from build123d import *

# Parameters (mm, degrees)
F0_W     = 3
F0_H     = 27
F1_DEPTH = 2


with BuildPart() as f1:
    # F0 (on Top) → F1 (new body)
    with BuildSketch(Plane.XY):
        with Locations((-86.87473, 11.051753)):
            Rectangle(F0_W, F0_H)
        with Locations((-82.87473, 11.051753)):
            Rectangle(F0_W, F0_H)
        with Locations((-78.87473, 11.051753)):
            Rectangle(F0_W, F0_H)
        with Locations((-74.87473, 11.051753)):
            Rectangle(F0_W, F0_H)
        with Locations((-70.87473, 11.051753)):
            Rectangle(F0_W, F0_H)
        with Locations((-66.87473, 11.051753)):
            Rectangle(F0_W, F0_H)
        with Locations((-62.87473, 11.051753)):
            Rectangle(F0_W, F0_H)
        with Locations((-58.87473, 11.051753)):
            Rectangle(F0_W, F0_H)
        with Locations((-54.87473, 11.051753)):
            Rectangle(F0_W, F0_H)
        with Locations((-50.87473, 11.051753)):
            Rectangle(F0_W, F0_H)
        with Locations((-46.87473, 11.051753)):
            Rectangle(F0_W, F0_H)
        with Locations((-42.87473, 11.051753)):
            Rectangle(F0_W, F0_H)
        with Locations((-38.87473, 11.051753)):
            Rectangle(F0_W, F0_H)
        with Locations((-34.87473, 11.051753)):
            Rectangle(F0_W, F0_H)
        with Locations((-30.87473, 11.051753)):
            Rectangle(F0_W, F0_H)
        with Locations((-26.87473, 11.051753)):
            Rectangle(F0_W, F0_H)
        with Locations((-22.87473, 11.051753)):
            Rectangle(F0_W, F0_H)
        with Locations((-18.87473, 11.051753)):
            Rectangle(F0_W, F0_H)
        with Locations((-14.87473, 11.051753)):
            Rectangle(F0_W, F0_H)
        with Locations((-10.87473, 11.051753)):
            Rectangle(F0_W, F0_H)
        with Locations((-6.87473, 11.051753)):
            Rectangle(F0_W, F0_H)
        with Locations((-2.87473, 11.051753)):
            Rectangle(F0_W, F0_H)
        with Locations((1.12527, 11.051753)):
            Rectangle(F0_W, F0_H)
        with Locations((5.12527, 11.051753)):
            Rectangle(F0_W, F0_H)
        with Locations((9.12527, 11.051753)):
            Rectangle(F0_W, F0_H)
        with Locations((13.12527, 11.051753)):
            Rectangle(F0_W, F0_H)
        with Locations((17.12527, 11.051753)):
            Rectangle(F0_W, F0_H)
        with Locations((21.12527, 11.051753)):
            Rectangle(F0_W, F0_H)
        with Locations((25.12527, 11.051753)):
            Rectangle(F0_W, F0_H)
        with Locations((29.12527, 11.051753)):
            Rectangle(F0_W, F0_H)
        with Locations((33.12527, 11.051753)):
            Rectangle(F0_W, F0_H)
        with Locations((37.12527, 11.051753)):
            Rectangle(F0_W, F0_H)
        with Locations((41.12527, 11.051753)):
            Rectangle(F0_W, F0_H)
        with Locations((45.12527, 11.051753)):
            Rectangle(F0_W, F0_H)
        with Locations((49.12527, 11.051753)):
            Rectangle(F0_W, F0_H)
        with Locations((53.12527, 11.051753)):
            Rectangle(F0_W, F0_H)
        with Locations((57.12527, 11.051753)):
            Rectangle(F0_W, F0_H)
        with Locations((61.12527, 11.051753)):
            Rectangle(F0_W, F0_H)
        with Locations((65.12527, 11.051753)):
            Rectangle(F0_W, F0_H)
        with Locations((69.12527, 11.051753)):
            Rectangle(F0_W, F0_H)
        with Locations((73.12527, 11.051753)):
            Rectangle(F0_W, F0_H)
        with Locations((77.12527, 11.051753)):
            Rectangle(F0_W, F0_H)
        with Locations((81.12527, 11.051753)):
            Rectangle(F0_W, F0_H)
        with Locations((85.12527, 11.051753)):
            Rectangle(F0_W, F0_H)
        Polygon((86.62527, 37.551753), (-88.37473, 37.551753), (-88.37473, 24.551753), (-85.37473, 24.551753), (-84.37473, 24.551753), (-81.37473, 24.551753), (-80.37473, 24.551753), (-77.37473, 24.551753), (-76.37473, 24.551753), (-73.37473, 24.551753), (-72.37473, 24.551753), (-69.37473, 24.551753), (-68.37473, 24.551753), (-65.37473, 24.551753), (-64.37473, 24.551753), (-61.37473, 24.551753), (-60.37473, 24.551753), (-57.37473, 24.551753), (-56.37473, 24.551753), (-53.37473, 24.551753), (-52.37473, 24.551753), (-49.37473, 24.551753), (-48.37473, 24.551753), (-45.37473, 24.551753), (-44.37473, 24.551753), (-41.37473, 24.551753), (-40.37473, 24.551753), (-37.37473, 24.551753), (-36.37473, 24.551753), (-33.37473, 24.551753), (-32.37473, 24.551753), (-29.37473, 24.551753), (-28.37473, 24.551753), (-25.37473, 24.551753), (-24.37473, 24.551753), (-21.37473, 24.551753), (-20.37473, 24.551753), (-17.37473, 24.551753), (-16.37473, 24.551753), (-13.37473, 24.551753), (-12.37473, 24.551753), (-9.37473, 24.551753), (-8.37473, 24.551753), (-5.37473, 24.551753), (-4.37473, 24.551753), (-1.37473, 24.551753), (-0.37473, 24.551753), (2.62527, 24.551753), (3.62527, 24.551753), (6.62527, 24.551753), (7.62527, 24.551753), (10.62527, 24.551753), (11.62527, 24.551753), (14.62527, 24.551753), (15.62527, 24.551753), (18.62527, 24.551753), (19.62527, 24.551753), (22.62527, 24.551753), (23.62527, 24.551753), (26.62527, 24.551753), (27.62527, 24.551753), (30.62527, 24.551753), (31.62527, 24.551753), (34.62527, 24.551753), (35.62527, 24.551753), (38.62527, 24.551753), (39.62527, 24.551753), (42.62527, 24.551753), (43.62527, 24.551753), (46.62527, 24.551753), (47.62527, 24.551753), (50.62527, 24.551753), (51.62527, 24.551753), (54.62527, 24.551753), (55.62527, 24.551753), (58.62527, 24.551753), (59.62527, 24.551753), (62.62527, 24.551753), (63.62527, 24.551753), (66.62527, 24.551753), (67.62527, 24.551753), (70.62527, 24.551753), (71.62527, 24.551753), (74.62527, 24.551753), (75.62527, 24.551753), (78.62527, 24.551753), (79.62527, 24.551753), (82.62527, 24.551753), (83.62527, 24.551753), (86.62527, 24.551753), align=None)
    extrude(amount=F1_DEPTH)


solid = f1.part
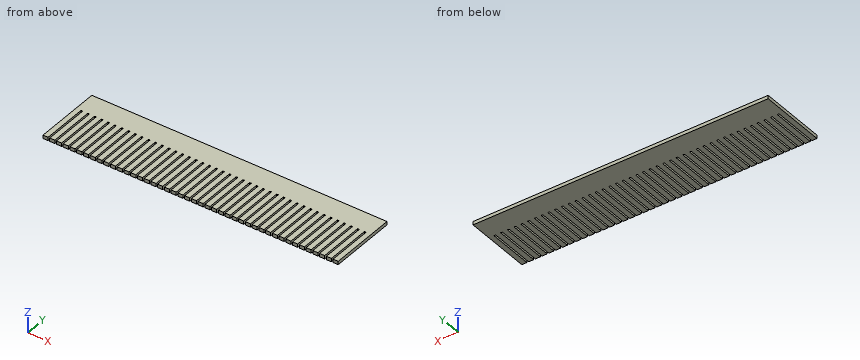
Model file for the job. Use its own axes, mm. Give positions to 0.01 mm unless a question says otherwise; leave off trailing zeros. Put each result on its own line as item: value. Start each with the question number.
(1) Band-saw the part on A-A on y = 1. Count the separate pieces of the cut face and the enclosed holes in it, then the cut area to 3 significant figures.
(2) Drill centre line: L1, parallel to Y at x = 3, z = 1.6. Where is it in solid material? Low to high. Write a range as [from, to].
(3) Pin check, flat tip, straight feed: pin 1 Ø0.5 at (x, z) = (-77, 0.5) entering from -Y. Stop position of the tip, or through.
Results below:
1. separate pieces: 44
1. enclosed holes: 0
1. area: 264 mm2
2. L1: y = [24.55, 37.55]
3. pin 1: stops at y = 24.55
